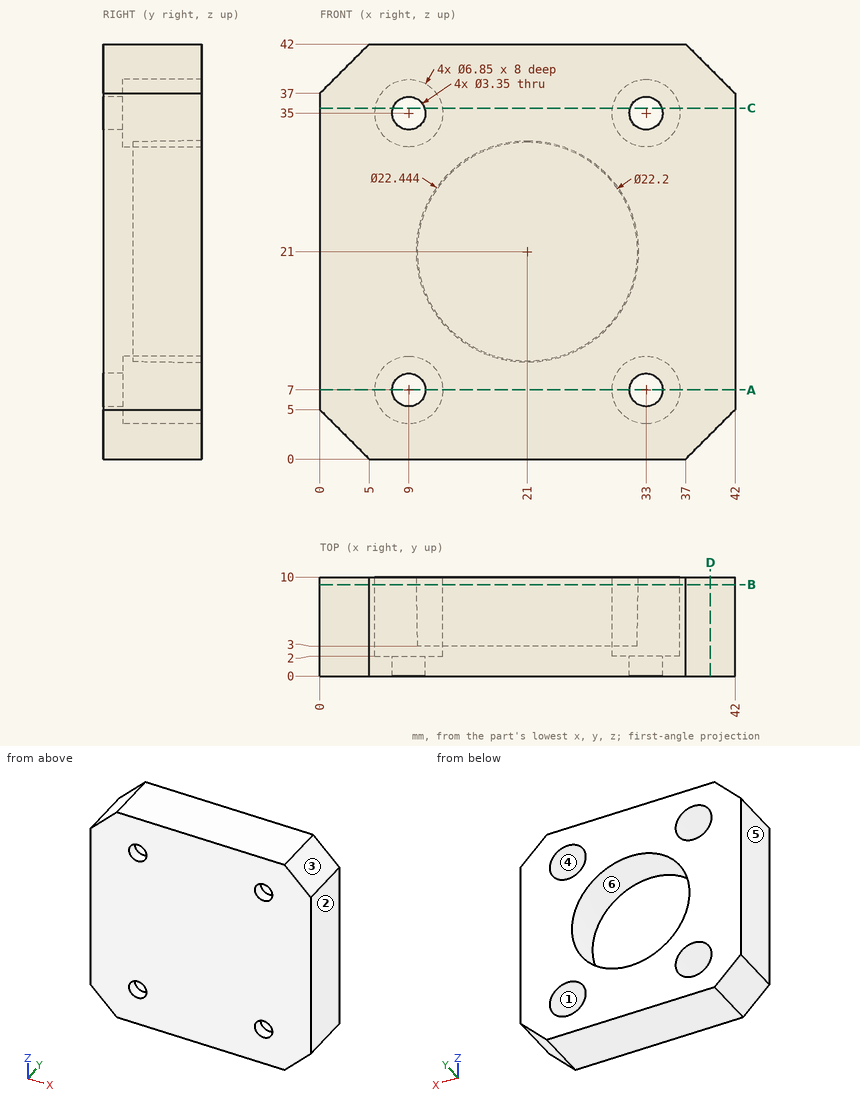
Check sheet for the drawn part. Datum: minimum x, y, z corner. Units: mm. A direction names the side the tool comes from. Round coordinates to 2 decimals unless told otherwise and drop trailing zeros. Order: outer loops, then holes, each group sorted by start corner. A loop starts at its lowest first (then second) coordinate and runs counter-clockwise, first axis right, second up. Notation, with made-up numbers: M -28.5,-18 L -20.5,-18 A23 cw -20.5,10 Z; hole C -34,-6 d8. An arc over 180 degrees is marked long. Answer in a Markdown table with one row per item.
(1) Section check A-A on z = 7. Record the boundary of the cut face in (x, y) (1 decimal), plus the area to 3 significant figures.
Findings:
| item | result |
|---|---|
| outline | M 0,0 L 7.3,0 L 7.3,2 L 5.6,2 L 5.6,10 L 0,10 Z; M 10.7,0 L 31.3,0 L 31.3,2 L 29.6,2 L 29.6,10 L 12.4,10 L 12.4,2 L 10.7,2 Z; M 34.7,0 L 42,0 L 42,10 L 36.4,10 L 36.4,2 L 34.7,2 Z |
| area | 297 mm^2 |
(2) Section check D-D on x = 39.5. Record the boundary of the cut face in (y, z), plus the area to 3 significant figures.
Findings:
| item | result |
|---|---|
| outline | M 0,2.5 L 10,2.5 L 10,39.5 L 0,39.5 Z |
| area | 370 mm^2 |
(3) Section check C-C on z = 35.5. Record the boundary of the cut face in (x, y), plus the area to 3 significant figures.
Findings:
| item | result |
|---|---|
| outline | M 0,0 L 7.4,0 L 7.4,2 L 5.61,2 L 5.61,10 L 0,10 Z; M 10.6,0 L 31.4,0 L 31.4,2 L 29.61,2 L 29.61,10 L 12.39,10 L 12.39,2 L 10.6,2 Z; M 34.6,0 L 42,0 L 42,10 L 36.39,10 L 36.39,2 L 34.6,2 Z |
| area | 299 mm^2 |
(4) Set-up check for the marked faces 1 and 2: record each of +Z, -Z, +X, -X, +Y, -Y from which the full face is reachable in a straight line by a thin tool's end or side.
Findings:
| item | result |
|---|---|
| face 1 | +Y |
| face 2 | +Z, -Z, +X, +Y, -Y |
(5) Draft check along Z on the marked faces 3, 4, 5 and 6. Enter one of: +Z half, -Z half, draft (parallel to the pull), parting line (faces both ways), or undercut.
Findings:
| item | result |
|---|---|
| face 3 | +Z half |
| face 4 | undercut |
| face 5 | draft |
| face 6 | undercut |
(6) Gauge pin test, flat ends, axial feed: pin 1 (11 mm diameter, centred on x = 23.5, z = 24.5, fed in from +Y); pin 2 (5.5 mm diameter, centred on x = 9, z = 7, fed in from +Y). Record the tip position at first contact, or that the pin passes through.
Findings:
| item | result |
|---|---|
| pin 1 | stops at y = 3 |
| pin 2 | stops at y = 2 |
(7) Material ranges on line 1 along X through (y, z) = (1.1, 7) (1 decimal); line 2 along X through (y, z) = (6.75, 35) (1 decimal); line 3 along Y through (x, z) = (20, 23), recorded low to high. Write a range as from..to.
Findings:
| item | result |
|---|---|
| line 1 | x = 0..7.3, 10.7..31.3, 34.7..42 |
| line 2 | x = 0..5.6, 12.4..29.6, 36.4..42 |
| line 3 | y = 0..3 |
(8) Section check B-B on y = 9.25. Give the number of separate pieces and of enclosed holes in the cut face, plus the area to 3 significant figures.
Findings:
| item | result |
|---|---|
| separate pieces | 1 |
| enclosed holes | 5 |
| area | 1,170 mm^2 |
